```python
from build123d import *

# Parameters (mm, degrees)
SKETCH1_W                    = 91
SKETCH1_H                    = 65
BOSS_EXTRUDE1_DEPTH          = 3
TAP_DRILL_FOR_M3X0_5_TAP1_D  = 2.5
FILLET1_R                    = 3
CSK_FOR_M3_SFHCS1_AT_2_COUNT = 2
CSK_FOR_M3_SFHCS1_AT_2_PITCH = 31.5
CSK_FOR_M3_SFHCS1_AT_3_COUNT = 2
CSK_FOR_M3_SFHCS1_AT_3_PITCH = 86.909435621
CSK_FOR_M3_SFHCS1_AT_4_COUNT = 2
CSK_FOR_M3_SFHCS1_AT_4_PITCH = 81


with BuildPart() as part:
    # Sketch1 → Boss-Extrude1 (new body)
    with BuildSketch(Plane.XY):
        Rectangle(SKETCH1_W, SKETCH1_H)
    extrude(amount=BOSS_EXTRUDE1_DEPTH)

    # Tap Drill for M3x0.5 Tap1 (through all)
    with Locations(Plane.XY.offset(3)):
        with Locations((-41.5, 28.5), (41.5, 28.5), (41.5, -28.5), (-41.5, -28.5)):
            Hole(TAP_DRILL_FOR_M3X0_5_TAP1_D / 2)

    # Fillet1
    fillet1_edges = [part.edges().sort_by_distance(p)[0] for p in [
        (-45.5, 32.5, 1.5),
        (45.5, 32.5, 1.5),
        (45.5, -32.5, 1.5),
        (-45.5, -32.5, 1.5),
    ]]
    fillet(fillet1_edges, radius=FILLET1_R)

    # Sketch7 → CSK for M3 SFHCS1 (revolve, cut)
    with BuildSketch(Plane(origin=(-40.5, 8, 3), x_dir=(0, -1, 0), z_dir=(1, 0, 0))):
        Polygon((0, 0), (0, 3), (1.6, 3), (1.6, 1.76), (3.36, 0), align=None)
    csk_for_m3_sfhcs1 = revolve(axis=Axis((-40.5, 8, 9.35), (0, 0, -1)), mode=Mode.SUBTRACT)

    # CSK for M3 SFHCS1 at 2: CSK for M3 SFHCS1 ×2
    with Locations(*[(0, -i * CSK_FOR_M3_SFHCS1_AT_2_PITCH, 0) for i in range(1, CSK_FOR_M3_SFHCS1_AT_2_COUNT)]):
        add(csk_for_m3_sfhcs1, mode=Mode.SUBTRACT)

    # CSK for M3 SFHCS1 at 3: CSK for M3 SFHCS1 ×2
    with Locations(*[Vector(0.932004671541296, -0.36244626115494855, 0) * (i * CSK_FOR_M3_SFHCS1_AT_3_PITCH) for i in range(1, CSK_FOR_M3_SFHCS1_AT_3_COUNT)]):
        add(csk_for_m3_sfhcs1, mode=Mode.SUBTRACT)

    # CSK for M3 SFHCS1 at 4: CSK for M3 SFHCS1 ×2
    with Locations(*[(i * CSK_FOR_M3_SFHCS1_AT_4_PITCH, 0, 0) for i in range(1, CSK_FOR_M3_SFHCS1_AT_4_COUNT)]):
        add(csk_for_m3_sfhcs1, mode=Mode.SUBTRACT)


solid = part.part
```
CAD build for the part. Positions are in the model's coordinates, mm. Coordinates: 2 decimals unless noted, no trailing zeros. Loops run counter-clockwise (first coordinate to the right, second up) from the corner with the lowest first, then second, coordinate; pieces in that order, holes last. Notation, with made-up numbers: (-12.75, -8.75) - (44.25, -8.75) arc R28 cw to (44.25, 27.25) - close; hole circle Ø11 at (78.25, 84). An arc over 180 degrees is marked (long way). Return JSON: item names as keys, results as strings.
1. Probe L1, parallel to X at y = -23.5, z = 0.75; L2, parallel to Y at x = 41.5, z = 1.15; L3, parallel to X at y = -28, z = 0.45. List the from-to ranges inside material, lowest first. Write a range as from..to.
Result:
{"L1": "x = -45.5..-42.1, -38.9..38.9, 42.1..45.5", "L2": "y = -32.5..-29.75, -27.25..-24.75, -22.25..6.75, 9.25..27.25, 29.75..32.5", "L3": "x = -45.5..-42.65, -40.35..40.35, 42.65..45.5"}
2. Band-saw the part on B-B (y = 8). Give the cut face in (x, z), and give its area (3 significant figures).
Result:
{"outline": "(-45.5, 0) - (-42.1, 0) - (-42.1, 1.24) - (-43.86, 3) - (-45.5, 3) - close; (-38.9, 0) - (38.9, 0) - (38.9, 1.24) - (37.14, 3) - (-37.14, 3) - (-38.9, 1.24) - close; (42.1, 0) - (45.5, 0) - (45.5, 3) - (43.86, 3) - (42.1, 1.24) - close", "area": "248 mm2"}
3. Mould opens along Y. For faces 1 (the flat face through (-45.5, 0, 1)), 2 (the cylindrical face through (-44.64, -31.6, 1.52)), 3 (the cylindrical face through (42.06, 8.35, 0.63)), 4 (the flat face through (-1, 32.5, 1)) say: released by +Y, released by -Y, zero draft, split by the parting line, or undercut.
Result:
{"face 1": "zero draft", "face 2": "released by -Y", "face 3": "undercut", "face 4": "released by +Y"}
4. Drop flat-ended pins along their axis: pin 1 (1.9 mm diameter, centred on x = -40.5, y = 8, fed in from +Z); pin 2 (4 mm diameter, centred on x = -40.5, y = -23.5, fed in from +Z). Give the stop position or say it passes through.
Result:
{"pin 1": "passes through", "pin 2": "stops at z = 1.64"}
5. Band-saw the part on A-A (y = 28.5). Give the cut face in (x, z).
Result:
{"outline": "(-45.5, 0) - (-42.75, 0) - (-42.75, 3) - (-45.5, 3) - close; (-40.25, 0) - (40.25, 0) - (40.25, 3) - (-40.25, 3) - close; (42.75, 0) - (45.5, 0) - (45.5, 3) - (42.75, 3) - close"}
6. Band-saw the part on C-C (y = -24). State how many separate pieces and enclosed holes the cut face has, and give its area (3 significant figures).
Result:
{"separate pieces": "3", "enclosed holes": "0", "area": "248 mm2"}
